Check sheet for the modelled part. Datum: model origin and axes. Units: mm. Give positions to 0.01 mm unless a question says otherwise; leave off trailing zeros. Write each loop counter-clockwise with the first axis right and the second up, starting at its lowest first coordinate (ties: lowest second). Pieces come first, ordered by that corner, then holes. Notation, with made-up numbers: (-25.75, 19.5) -> (-2.75, 19.5) arc R20 cw to (-2.75, 28.5) -> close; hole circle Ø5 at (11, 41.5). An arc over 180 degrees is marked (long way). Return JSON: item names as keys, results as strings.
from build123d import *

# Parameters (mm, degrees)
SKETCH2_W            = 45
SKETCH2_H            = 53.556000076
BOSS_EXTRUDE1_DEPTH  = 1.5
M3_CLEARANCE_HOLE_D  = 3.4
M3_CLEARANCE_HOLE1_D = 3.4
CUT_EXTRUDE1_REACH   = 37.008
SKETCH17_R           = 4.445


with BuildPart() as part:
    # Sketch2 → Boss-Extrude1 (new body)
    with BuildSketch(Plane(origin=(0, 0, 0), x_dir=(1, 0, 0), z_dir=(0, 1, 0))):
        Rectangle(SKETCH2_W, SKETCH2_H)
    extrude(amount=BOSS_EXTRUDE1_DEPTH)

    # M3 Clearance Hole (through all)
    with Locations(Plane(origin=(0, 1.5, 0), x_dir=(1, 0, 0), z_dir=(0, 1, 0))):
        with Locations((-15.736599944, 20), (15, 20), (15, -20), (-15.736599944, -20), (0, 0)):
            Hole(M3_CLEARANCE_HOLE_D / 2)

    # M3 Clearance Hole1 (through all)
    with Locations(Plane(origin=(0, 1.5, 0), x_dir=(1, 0, 0), z_dir=(0, 1, 0))):
        with Locations((-8.838834765, -8.838834765), (-8.838834765, 8.838834765), (8.838834765, -8.838834765), (8.838834765, 8.838834765)):
            Hole(M3_CLEARANCE_HOLE1_D / 2)

    # Sketch17 → Cut-Extrude1 (cut, up to next)
    with BuildSketch(Plane(origin=(0, 1.5, 0), x_dir=(1, 0, 0), z_dir=(0, 1, 0)), mode=Mode.PRIVATE) as cut_extrude1_sk1:
        with Locations(Location((0, 0, 0), (0, 0, 270))):
            Circle(SKETCH17_R)
    cut_extrude1_tool1 = extrude(cut_extrude1_sk1.sketch, amount=-CUT_EXTRUDE1_REACH, mode=Mode.PRIVATE) & part.part
    add(cut_extrude1_tool1.solids().sort_by_distance((0, 1.5, 0))[0], mode=Mode.SUBTRACT)


solid = part.part
(1) Release check for a two-part mould opening along X. For faces 1 (the cylindrical face through (13.38, 0.74, -20.51)), 2 (the flat face through (5, 0, 0)), 3 (the flat face through (-22.5, 1, 0)), 4 (the cylindrical face through (10.19, 0.74, 9.87)) record: pulls with the +X half, pulls with the -X half, needs draft (parallel to the pull), parting line crosses it, or undercut.
Reply:
{"face 1": "undercut", "face 2": "needs draft", "face 3": "pulls with the -X half", "face 4": "undercut"}
(2) Cross-section at B-B on x = 0. Enter the section's corners in (y, z) (3 decimals).
Reply:
{"outline": "(0, -26.778) -> (1.5, -26.778) -> (1.5, -4.445) -> (0, -4.445) -> close; (0, 4.445) -> (1.5, 4.445) -> (1.5, 26.778) -> (0, 26.778) -> close"}
(3) Cross-section at C-C on z = 0. Enter the section's corners in (x, y) (3 decimals).
Reply:
{"outline": "(-22.5, 0) -> (-4.445, 0) -> (-4.445, 1.5) -> (-22.5, 1.5) -> close; (4.445, 0) -> (22.5, 0) -> (22.5, 1.5) -> (4.445, 1.5) -> close"}
(4) Depth check by flat-ended pin: pin 1 Ø2.5 at (x, z) = (8.84, -8.84) entering from -Y. Enter the tip coordinate at first touch or a pass-through.
Reply:
{"pin 1": "through"}
(5) Thickness scan on L1, parallel to X at y = 0.6, z = 20; L2, parallel to X at y = 0.5, z = 10; L3, parallel to Z at x = -15, y = 0.9. Record the ranges inside material, lowest first.
Reply:
{"L1": "-22.5 to -17.44, -14.04 to 13.3, 16.7 to 22.5", "L2": "-22.5 to -10.08, -7.6 to 7.6, 10.08 to 22.5", "L3": "-26.78 to -21.53, -18.47 to 18.47, 21.53 to 26.78"}
(6) Cross-section at D-D on y = 0.25. State how many separate pieces and enclosed holes the cut face has, then the cut area to 3 significant figures.
Reply:
{"separate pieces": "1", "enclosed holes": "9", "area": "2,280 mm^2"}
(7) Cross-section at A-A on x = 15. Enter the section's corners in (y, z), then the cut area to 3 significant figures.
Reply:
{"outline": "(0, -26.78) -> (1.5, -26.78) -> (1.5, -21.7) -> (0, -21.7) -> close; (0, -18.3) -> (1.5, -18.3) -> (1.5, 18.3) -> (0, 18.3) -> close; (0, 21.7) -> (1.5, 21.7) -> (1.5, 26.78) -> (0, 26.78) -> close", "area": "70.1 mm^2"}
